Could you check a few things on this model? Use its own coordinates, in mm. Face numbers are marked on the shaded views. A direction names the side the tool comes from. Coordinates: 2 decimals unless noted, no trailing zeros. Loops run counter-clockwise (first coordinate to the right, second up) from the corner with the lowest first, then second, coordinate; pieces in that order, holes last. Notation, with made-up numbers: (13.5, 0) - (65.5, 0) arc R37 ccw to (65.5, 36) - close; hole circle Ø4 at (40.5, 53). An arc over 180 degrees is marked (long way). One line per question, with ' | ' between items. Start each with the question number.
1. I want a section at B-B, the plane y = 20. Write out the boundary of the cut face in (x, z).
2. I'm going to push flat-ended pins straight in: P1, Ø1, axis at x = 94.5, y = 9.5, coming from the -Z side; P2, Ø2, axis at x = 82.5, z = 16.5, coming from the +Y side; P3, Ø1, axis at x = 44, z = 24, coming from the -Y side; P4, Ø5, axis at x = 26, z = 11.5, coming from the -Y side. Where does each tip first touch, or does it pass through?
3. I want a section at D-D, the plane x = 38.5. Write out the boundary of the cut face in (y, z), then the cut area to 3 significant figures.
4. I want a section at C-C, the plane z = 21. Write out the boundary of the cut face in (x, y).
5. I want a section at A-A, the plane x = 61.5. Write out the boundary of the cut face in (y, z), then the cut area to 3 significant figures.
6. Please list where these lines run through material, in increasing order: L1, parallel to Y at x = 30, z = 9.75; L2, parallel to X at y = 20, z = 10.5; L3, parallel to X at y = 70, z = 8.5. Write a range as [from, to].
7. Which directions (+Z, -Z, +X, -X, +Y, -Y) give clear straight access to the entire face, cutting with the end or side of a thin tool? Please do the marked faces 5 and 6.
8. We'd pull the mould along Y, two halves only. Please class the marked faces 1, 2, 3 and 4: pulls with the +Y half, pulls with the -Y half, needs draft (parallel to the pull), parting line crosses it, or undercut.
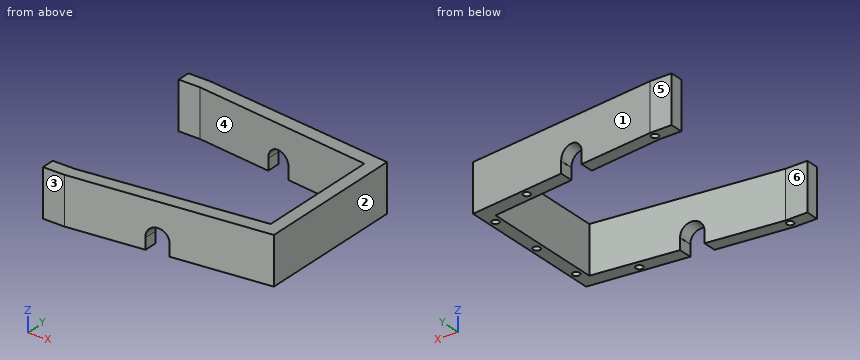
from build123d import *

# Parameters (mm, degrees)
SKETCH044_W      = 10.390858
SKETCH044_H      = 5.392216
EXTRUDE047_DEPTH = 100
SKETCH179_R      = 1.623797
EXTRUDE196_DEPTH = 10
SKETCH178_R      = 5.177463
EXTRUDE195_DEPTH = 800
EXTRUDE194_DEPTH = 22


with BuildPart() as extrude047:
    # Sketch044 → Extrude047 (new body)
    with BuildSketch(Plane.XZ):
        with Locations((70, -7.3389)):
            Rectangle(SKETCH044_W, SKETCH044_H)
    extrude(amount=EXTRUDE047_DEPTH)


with BuildPart() as extrude047_1:
    # Extrude047 placement: moved
    add(extrude047.part.moved(Location((0, 96.2, 0))))


with BuildPart() as extrude196:
    # Sketch179 → Extrude196 (new body)
    with BuildSketch(Plane.XY.offset(12.1)):
        with Locations((30, 86.963425)):
            Circle(SKETCH179_R)
        with Locations((30, 3.252438)):
            Circle(SKETCH179_R)
        with Locations((95.163345, 10)):
            Circle(SKETCH179_R)
        with Locations((94.949776, 80)):
            Circle(SKETCH179_R)
        with Locations((117.10096, 20)):
            Circle(SKETCH179_R)
        with Locations((117.030609, 70)):
            Circle(SKETCH179_R)
        with Locations((117.10096, 44.443623)):
            Circle(SKETCH179_R)
    extrude(amount=EXTRUDE196_DEPTH)


with BuildPart() as extrude196_1:
    # Extrude196 placement: moved
    add(extrude196.part.moved(Location((0, 0, -24.5))))


with BuildPart() as extrude195:
    # Sketch178 → Extrude195 (new body)
    with BuildSketch(Plane.XZ):
        with Locations((70, 3.62)):
            Circle(SKETCH178_R)
    extrude(amount=EXTRUDE195_DEPTH)


with BuildPart() as extrude195_1:
    # Extrude195 placement: moved
    add(extrude195.part.moved(Location((0, 293, 0))))


with BuildPart() as obj1:
    # Sketch177 → Extrude194 (new body)
    with BuildSketch(Plane.XY):
        Polygon((30, 0), (120, 10), (120, 80), (30, 90), (20, 90), (20, 84), (30, 84), (114, 74), (114, 16), (30.22679, 6), (20, 6), (20, 0), align=None)
    extrude(amount=EXTRUDE194_DEPTH)


with BuildPart() as obj1_1:
    # Extrude194 placement: moved
    add(obj1.part.moved(Location((0, 0, -2))))

    # Cut123: cut Extrude195
    add(extrude195_1.part, mode=Mode.SUBTRACT)


with BuildPart() as obj1_2:
    # Cut123 placement: moved
    add(obj1_1.part.moved(Location((0, 0, -7.9))))

    # Cut015: cut Extrude196
    add(extrude196_1.part, mode=Mode.SUBTRACT)

    # Cut016: cut Extrude047
    add(extrude047_1.part, mode=Mode.SUBTRACT)


with BuildPart() as obj1_3:
    # Cut016 placement: moved
    add(obj1_2.part.moved(Location((0, 0, 15.75))))


solid = obj1_3.part
Results are:
1) outline: (114, 5.85) - (115.48, 5.85) - (115.48, 13.35) - (118.72, 13.35) - (118.72, 5.85) - (120, 5.85) - (120, 27.85) - (114, 27.85) - close
2) P1: stops at z = 13.35 | P2: stops at y = 84.28 | P3: stops at y = 1.5 | P4: stops at y = 0
3) outline: (0.94, 5.85) - (6.99, 5.85) - (6.99, 27.85) - (0.94, 27.85) - close; (82.99, 5.85) - (89.06, 5.85) - (89.06, 27.85) - (82.99, 27.85) - close | area: 266 mm2
4) outline: (20, 0) - (30, 0) - (120, 10) - (120, 80) - (30, 90) - (20, 90) - (20, 84) - (30, 84) - (114, 74) - (114, 16) - (30.23, 6) - (20, 6) - close
5) outline: (3.5, 5.85) - (9.73, 5.85) - (9.73, 27.85) - (3.5, 27.85) - close; (80.25, 5.85) - (86.5, 5.85) - (86.5, 27.85) - (80.25, 27.85) - close | area: 275 mm2
6) L1: y = [0, 1.63], [4.88, 6], [84, 85.34], [88.59, 90] | L2: x = [114, 115.48], [118.72, 120] | L3: x = [114, 115.41], [118.65, 120]
7) face 5: +Z, -Z, +X, -X, +Y | face 6: +Z, -Z, -X
8) face 1: pulls with the +Y half | face 2: needs draft | face 3: pulls with the -Y half | face 4: undercut
